```python
from build123d import *

# Parameters (mm, degrees)
BOSS_EXTRUDE4_DEPTH = 17
SKETCH3_R           = 8.25
CUT_EXTRUDE1_DEPTH  = 7
CUT_EXTRUDE2_START  = -7
SKETCH4_R           = 8.25
CUT_EXTRUDE2_DEPTH  = 7
CUT_EXTRUDE3_DEPTH  = 127.783772621
SKETCH6_R           = 5
CUT_EXTRUDE4_DEPTH  = 16.6
FILLET1_R           = 3


with BuildPart() as part:
    # Sketch2 → Boss-Extrude4 (new body)
    with BuildSketch(Plane.XY):
        with BuildLine():
            Line((-100, 10.25), (0, 10.25))
            ThreePointArc((0, 10.25), (10.25, 0), (0, -10.25))
            Line((0, -10.25), (-100, -10.25))
            ThreePointArc((-100, -10.25), (-110.25, 0), (-100, 10.25))
        make_face()
        with BuildLine():
            Line((-7.247844507, -7.247844507), (-57.247844507, 42.752155493))
            ThreePointArc((-57.247844507, 42.752155493), (-57.247844507, 57.247844507), (-42.752155493, 57.247844507))
            Line((-42.752155493, 57.247844507), (7.247844507, 7.247844507))
            ThreePointArc((7.247844507, 7.247844507), (7.247844507, -7.247844507), (-7.247844507, -7.247844507))
        make_face()
        with BuildLine():
            Line((-107.247844507, 7.247844507), (-57.247844507, 57.247844507))
            ThreePointArc((-57.247844507, 57.247844507), (-42.752155493, 57.247844507), (-42.752155493, 42.752155493))
            Line((-42.752155493, 42.752155493), (-92.752155493, -7.247844507))
            ThreePointArc((-92.752155493, -7.247844507), (-107.247844507, -7.247844507), (-107.247844507, 7.247844507))
        make_face()
    extrude(amount=BOSS_EXTRUDE4_DEPTH)

    # Sketch3 → Cut-Extrude1 (cut)
    with BuildSketch(Plane(origin=(0, 0, 0), x_dir=(-1, 0, 0), z_dir=(0, 0, -1))):
        Circle(SKETCH3_R)
        with Locations((50, 50)):
            Circle(SKETCH3_R)
        with Locations((100, 0)):
            Circle(SKETCH3_R)
    extrude(amount=-CUT_EXTRUDE1_DEPTH, mode=Mode.SUBTRACT)

    # Sketch4 → Cut-Extrude2 (cut)
    with BuildSketch(Plane.XY.offset(17).offset(CUT_EXTRUDE2_START)):
        with Locations(Location((-100, 0, 0), (0, 0, 180))):
            Circle(SKETCH4_R)
        with Locations(Location((-50, 50, 0), (0, 0, 180))):
            Circle(SKETCH4_R)
        with Locations(Location((0, 0, 0), (0, 0, 180))):
            Circle(SKETCH4_R)
    extrude(amount=CUT_EXTRUDE2_DEPTH, mode=Mode.SUBTRACT)

    # Sketch5 → Cut-Extrude3 (cut, through all)
    with BuildSketch(Plane(origin=(0, 0, 0), x_dir=(-1, 0, 0), z_dir=(0, 0, -1))):
        Polygon((17.5, 8.25), (50, 40.75), (82.5, 8.25), align=None)
    extrude(amount=-CUT_EXTRUDE3_DEPTH, mode=Mode.SUBTRACT)

    # Sketch6 → Cut-Extrude4 (cut)
    with BuildSketch(Plane.XY.offset(17)):
        with Locations((-100, 0)):
            Circle(SKETCH6_R)
        with Locations((-50, 50)):
            Circle(SKETCH6_R)
        Circle(SKETCH6_R)
    extrude(amount=-CUT_EXTRUDE4_DEPTH, mode=Mode.SUBTRACT)

    # Fillet1
    fillet1_edges = [part.edges().sort_by_distance(p)[0] for p in [
        (-82.5, 8.25, 8.5),
        (-17.5, 8.25, 8.5),
        (-50, 40.75, 8.5),
    ]]
    fillet(fillet1_edges, radius=FILLET1_R)


solid = part.part
```
Read the model definition and answer for the solid it produces. Units are mm, in the model's axes. A direction names the side the tool comes from. Give positions to 0.01 mm unless a question says otherwise; leave off trailing zeros. Write each loop counter-clockwise with the first axis right and the second up, starting at its lowest first coordinate (ties: lowest second). Pieces come first, ordered by that corner, then holes. Notation, with made-up numbers: M 22,76 L 79,76 A21 ccw 79,100 Z; hole C 66,8 d2. An arc over 180 degrees is marked long. Put each result on its own line as item: value. Start each with the question number.
1. Which of the six approach directions +Z, -Z, +X, -X, +Y, -Y give full straight-line access (tool end or side, diameter ignored) to faces 1 (the cylindrical face through (-7.62, -3.16, 3.45)), 2 (the flat face through (-35.07, 25.82, 8.38)), 3 (the cylindrical face through (-109.404, -4.078, 8.381)), 4 (the flat face through (-104, 4, 10))?
2. The part is cut by section D-D, the plane x = -103. Give the vertices of the cut face in (y, z), and give its area (3 significant figures).
3. For a pull along Y with two mould halves and no side action, classify faces 5 (the flat face through (-4, 4, 10)), 6 (the cylindrical face through (9.53, -3.77, 8.38)), 7 (the flat face through (-82.598, 31.898, 8.381)) as released by +Y, released by -Y, zero draft, split by the parting line, or undercut.
4. Each of these flat-tipped pins is pushed along its axis until it touches: pin 1 Ø6 at (y, z) = (8, 13.5) entering from -X; pin 2 Ø2 at (x, z) = (-26.5, 14.5) entering from +Y; pin 3 Ø1.5 at (y, z) = (9, 7.5) entering from +X; pin 4 Ø5 at (x, y) = (-98, -1) entering from -Z. Where does it stop, or does it pass through?
5. The part is cut by section A-A, the plane y = 0. Give the vertices of the cut face in (x, z), and give its area (3 significant figures).
6. Consider line 1 along Y through (x, z) = (-53, 2.75); line 2 along Y through (x, z) = (-42.5, 6.25); line 3 along X through (y, z) = (-6, 13.75). Determine where each line is inside the solid, lowest interval first.
7. The part is cut by section B-B, the plane z = 15.25. Give the vertices of the cut face in (x, y).
8. The part is cut by section C-C, the plane y = 24.5. Give the vertices of the cut face in (x, z).
Final values:
1. face 1: -Z
1. face 2: +Z, -Z
1. face 3: +Z, -Z, -X
1. face 4: +Z
2. outline: M -9.8,0 L -7.69,0 L -7.69,7 L -4,7 L -4,10 L -7.69,10 L -7.69,17 L -9.8,17 Z; M 4,7 L 7.69,7 L 7.69,0 L 11.5,0 L 11.5,17 L 7.69,17 L 7.69,10 L 4,10 Z
2. area: 123 mm²
3. face 5: undercut
3. face 6: split by the parting line
3. face 7: released by +Y
4. pin 1: stops at x = -108.95
4. pin 2: stops at y = 42
4. pin 3: stops at x = 6.25
4. pin 4: passes through
5. outline: M -110.25,0 L -108.25,0 L -108.25,7 L -105,7 L -105,10 L -108.25,10 L -108.25,17 L -110.25,17 Z; M -95,7 L -91.75,7 L -91.75,0 L -8.25,0 L -8.25,7 L -5,7 L -5,10 L -8.25,10 L -8.25,17 L -91.75,17 L -91.75,10 L -95,10 Z; M 5,7 L 8.25,7 L 8.25,0 L 10.25,0 L 10.25,17 L 8.25,17 L 8.25,10 L 5,10 Z
5. area: 1,530 mm²
6. line 1: y = -10.25 to 8.25, 37.75 to 42.31, 57.69 to 59.8
6. line 2: y = -10.25 to 8.25, 33.25 to 46.56, 53.44 to 57
6. line 3: x = -108.31 to -105.66, -94.34 to -5.66, 5.66 to 8.31
7. outline: M -107.25,7.25 A10.25 ccw -100,-10.25 L 0,-10.25 A10.25 ccw 7.25,7.25 L -42.75,57.25 A10.25 ccw -57.25,57.25 Z; hole C -100,0 d16.5; hole M -77.38,13.37 A3 ccw -75.26,8.25 L -24.74,8.25 A3 ccw -22.62,13.37 L -47.88,38.63 A3 ccw -52.12,38.63 Z; hole C -50,50 d16.5; hole C 0,0 d16.5
8. outline: M -90,0 L -66.25,0 L -66.25,17 L -90,17 Z; M -33.75,0 L -10,0 L -10,17 L -33.75,17 Z
